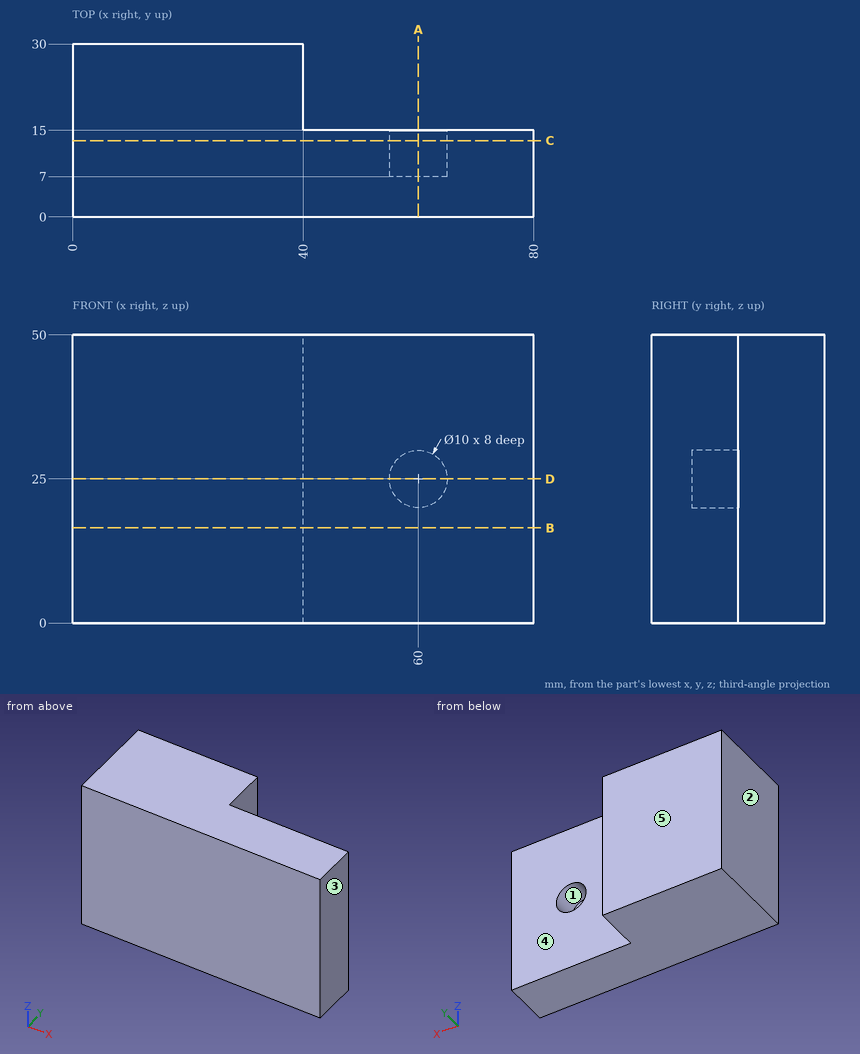
Could you check a few things on this drawing? It's one solid part, dimensions in mm from its lowest x, y, z. A direction names the side the tool comes from. Give positions to 0.01 mm unless a question says otherwise; leave off trailing zeros. Order: outer loops, then holes, each group sorted by start corner. A loop starts at its lowest first (then second) coordinate and runs counter-clockwise, first axis right, second up. Notation, with made-up numbers: (42, 81) - (58, 81) arc R10 cw to (58, 87) - close; hole circle Ø5 at (48, 30.25). An arc over 180 degrees is marked (long way). One line per item, written item: value. Start each with the question number.
1. Thinking about a two-plate mould opening in X: for the marked faces 1, 2 and 3, which applies, +X half, -X half, draft (parallel to the pull), parting line (faces both ways), or undercut?
2. For the marked faces 4 and 5, which set-ups out of +Z, -Z, +X, -X, +Y, -Y let a thin tool reach every point of the face, with its end or its side?
3. Imagine slicing it at A-A on x = 60. List the corners of the cut face in (y, z) for me, plus the area to 3 significant figures.
4. Imagine slicing it at C-C on y = 13.25. List the corners of the cut face in (x, z) for me, plus the area to 3 significant figures.
5. For P1, Ø10, axis at y = 22.5, z = 38.5, coming from the +X side; P2, Ø12, axis at x = 58.5, z = 35.5, coming from the +Y side; P3, Ø3, axis at x = 57.5, z = 27, coming from the +Y side, each with a flat end and sliding along its axis, tell me the tip position at first contact or that it passes through.
6. Imagine slicing it at B-B on z = 16.5. List the corners of the cut face in (x, y) for me.
7. If I drill on probe 1 along X at (y, z) = (13.5, 25); probe 2 along Y at (x, z) = (60, 37.5); probe 3 along X at (y, z) = (16, 10), over which ranges is the centre line in solid material (lowest first)?
8. Imagine slicing it at D-D on z = 25. List the corners of the cut face in (x, y) for me, plus the area to 3 significant figures.
Values:
1. face 1: undercut
1. face 2: -X half
1. face 3: +X half
2. face 4: +Z, -Z, +X, +Y
2. face 5: +Z, -Z, +X, -X, +Y
3. outline: (0, 0) - (15, 0) - (15, 20) - (7, 20) - (7, 30) - (15, 30) - (15, 50) - (0, 50) - close
3. area: 670 mm²
4. outline: (0, 0) - (80, 0) - (80, 50) - (0, 50) - close; hole circle Ø10 at (60, 25)
4. area: 3,920 mm²
5. P1: x = 40
5. P2: y = 15
5. P3: y = 7
6. outline: (0, 0) - (80, 0) - (80, 15) - (40, 15) - (40, 30) - (0, 30) - close
7. probe 1: 0 to 55, 65 to 80
7. probe 2: 0 to 15
7. probe 3: 0 to 40
8. outline: (0, 0) - (80, 0) - (80, 15) - (65, 15) - (65, 7) - (55, 7) - (55, 15) - (40, 15) - (40, 30) - (0, 30) - close
8. area: 1,720 mm²
